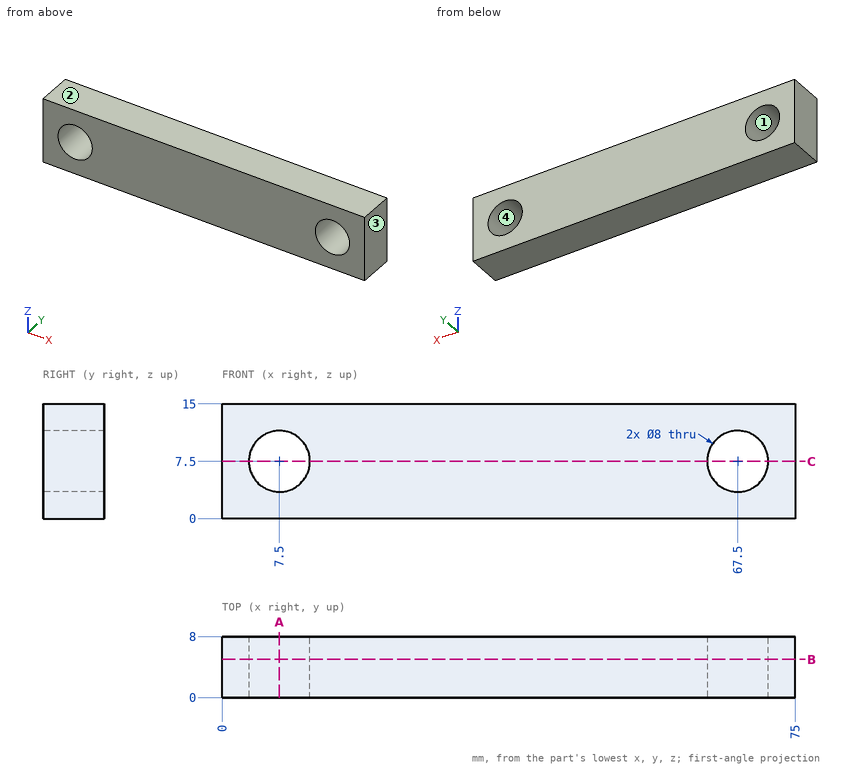
Answer from the drawing. Dimensions are ordinates in mm from the lowest x, y and z of the part. Coordinates: 2 decimals unless noted, no trailing zeros. Order: outer loops, then holes, each group sorted by start corner. A loop starts at its lowest first (then second) coordinate and runs counter-clockwise, first axis right, second up. Notation, with made-up numbers: (80.25, 87) -> (119.25, 87) arc R25 ccw to (119.25, 111) -> close; hole circle Ø6 at (57.25, 32). An arc over 180 degrees is marked (long way). Answer as a JSON object with one key per item and string values.
1) A cutting plane is placed at A-A, the plane x = 7.5. Determine the outline of the cut face in (y, z).
Model answer:
{"outline": "(0, 0) -> (8, 0) -> (8, 3.5) -> (0, 3.5) -> close; (0, 11.5) -> (8, 11.5) -> (8, 15) -> (0, 15) -> close"}
2) The mould has two halves that part along Z. Classify the marked faces 1, 2, 3 and 4: released by +Z, released by -Z, zero draft, split by the parting line, or undercut.
Model answer:
{"face 1": "undercut", "face 2": "released by +Z", "face 3": "zero draft", "face 4": "undercut"}
3) Consider line 1 along Z through (x, y) = (67.5, 4.25); line 2 along X through (y, z) = (4, 4.25); line 3 along X through (y, z) = (4.25, 6). Determine where each line is inside the solid, lowest interval first. Write a range as from..to.
Model answer:
{"line 1": "z = 0..3.5, 11.5..15", "line 2": "x = 0..5.17, 9.83..65.17, 69.83..75", "line 3": "x = 0..3.79, 11.21..63.79, 71.21..75"}
4) A cutting plane is placed at B-B, the plane y = 5. Determine the outline of the cut face in (x, z).
Model answer:
{"outline": "(0, 0) -> (75, 0) -> (75, 15) -> (0, 15) -> close; hole circle Ø8 at (7.5, 7.5); hole circle Ø8 at (67.5, 7.5)"}
5) A cutting plane is placed at C-C, the plane z = 7.5. Determine the outline of the cut face in (x, y), plus the area to 3 significant figures.
Model answer:
{"outline": "(0, 0) -> (3.5, 0) -> (3.5, 8) -> (0, 8) -> close; (11.5, 0) -> (63.5, 0) -> (63.5, 8) -> (11.5, 8) -> close; (71.5, 0) -> (75, 0) -> (75, 8) -> (71.5, 8) -> close", "area": "472 mm²"}
